```python
from build123d import *

# Parameters (mm, degrees)
SKETCH1_W           = 360
SKETCH1_H           = 210
BOSS_EXTRUDE1_DEPTH = 1
SKETCH2_R           = 5
SKETCH2_R_2         = 2.3
BOSS_EXTRUDE2_DEPTH = 5.7


with BuildPart() as part:
    # Sketch1 → Boss-Extrude1 (new body)
    with BuildSketch(Plane(origin=(0, 0, 0), x_dir=(1, 0, 0), z_dir=(0, 1, 0))):
        Rectangle(SKETCH1_W, SKETCH1_H)
        Polygon((28, -45.5), (0, -45.5), (0, 45.5), (-78.4, 45.5), (-78.4, -7.9), (-95, -7.9), (-95, 79.1), (-78.4, 79.1), (-78.4, 68.1), (28, 68.1), (28, 45.5), (66.5, 45.5), (66.5, -45.5), (66.5, -97), (28, -97), align=None, mode=Mode.SUBTRACT)
    extrude(amount=BOSS_EXTRUDE1_DEPTH)

    # Sketch2 → Boss-Extrude2 (add)
    with BuildSketch(Plane(origin=(0, 1, 0), x_dir=(1, 0, 0), z_dir=(0, 1, 0))):
        with Locations((-71.4, 75.1)):
            Circle(SKETCH2_R)
        with Locations((-71.4, 75.1)):
            Circle(SKETCH2_R_2, mode=Mode.SUBTRACT)
        with Locations((-71.4, 38.5)):
            Circle(SKETCH2_R)
        with Locations((-71.4, 38.5)):
            Circle(SKETCH2_R_2, mode=Mode.SUBTRACT)
        with Locations((-102, 75.1)):
            Circle(SKETCH2_R)
        with Locations((-102, 75.1)):
            Circle(SKETCH2_R_2, mode=Mode.SUBTRACT)
        with Locations((-7, 38.5)):
            Circle(SKETCH2_R)
        with Locations((-7, 38.5)):
            Circle(SKETCH2_R_2, mode=Mode.SUBTRACT)
        with Locations((35, 52.5)):
            Circle(SKETCH2_R)
        with Locations((35, 52.5)):
            Circle(SKETCH2_R_2, mode=Mode.SUBTRACT)
        with Locations((21, -52.5)):
            Circle(SKETCH2_R)
        with Locations((21, -52.5)):
            Circle(SKETCH2_R_2, mode=Mode.SUBTRACT)
        with Locations((-71.4, -0.9)):
            Circle(SKETCH2_R)
        with Locations((-71.4, -0.9)):
            Circle(SKETCH2_R_2, mode=Mode.SUBTRACT)
        with Locations((-102, -0.9)):
            Circle(SKETCH2_R)
        with Locations((-102, -0.9)):
            Circle(SKETCH2_R_2, mode=Mode.SUBTRACT)
        with Locations((73.5, 38.5)):
            Circle(SKETCH2_R)
        with Locations((73.5, 38.5)):
            Circle(SKETCH2_R_2, mode=Mode.SUBTRACT)
        with Locations((73.5, -90)):
            Circle(SKETCH2_R)
        with Locations((73.5, -90)):
            Circle(SKETCH2_R_2, mode=Mode.SUBTRACT)
        with Locations((21, -90)):
            Circle(SKETCH2_R)
        with Locations((21, -90)):
            Circle(SKETCH2_R_2, mode=Mode.SUBTRACT)
    extrude(amount=BOSS_EXTRUDE2_DEPTH)


solid = part.part
```
Model file for the job. Use its own axes, mm. A direction names the side the tool comes from. Round coordinates to 2 decimals unless told otherwise and drop trailing zeros. Write each loop counter-clockwise with the first axis right and the second up, starting at its lowest first coordinate (ties: lowest second). Pieces come first, ordered by that corner, then holes. Notation, with made-up numbers: (28, -23) -> (68, -23) arc R26 ccw to (68, -6) -> close; hole circle Ø2 at (-19.5, 63). An arc over 180 degrees is marked (long way). Answer as CSV lines item,"result".
1. Mould opens along X. For faces 3 (the face through (76.188, 3.81, -42.716)), 4 (the face through (-6, 6.7, -36)), 5 (the face through (31.315, 3.81, -55.879)) say: +X half, -X half, draft (parallel to the pull), parting line (faces both ways), or undercut.
Resolved:
face 3,"undercut"
face 4,"draft"
face 5,"parting line"
2. Tool access for faces 1 (the face through (-66.781, 3.81, 2.815)), 2 (the face through (76, 6.7, 91)): list every direction of +Z, -Z, +X, -X, +Y, -Y with a clear straight run to the whole face (end or side of a thin tool).
Resolved:
face 1,"+Y"
face 2,"+Z, -Z, +X, -X, +Y"
3. Drill centre lines: line 1 (Z direction, x = 73.5, y = 5.45); line 2 (X direction, y = 3.25, z = -38.5); line 3 (X direction, y = 2.8, z = -75.1). Where is each one in solid material? Low to high.
Resolved:
line 1,"-43.5 to -40.8, -36.2 to -33.5, 85 to 87.7, 92.3 to 95"
line 2,"-76.4 to -73.7, -69.1 to -66.4, -12 to -9.3, -4.7 to -2, 68.5 to 71.2, 75.8 to 78.5"
line 3,"-107 to -104.3, -99.7 to -97, -76.4 to -73.7, -69.1 to -66.4"
4. Slice it at A-A, the plane z = -63. List the corners of the cut face in (x, y), plus the area to 3 significant figures.
Resolved:
outline,"(-180, 0) -> (-95, 0) -> (-95, 1) -> (-180, 1) -> close; (28, 0) -> (180, 0) -> (180, 1) -> (28, 1) -> close"
area,"237 mm²"
5. Pin check, flat tips, straight feed: pin 1 Ø1 at (x, z) = (-110.5, 55.5) entering from +Y; pin 2 Ø2 at (y, z) = (2.5, 17.5) entering from +X; pin 3 Ø1.5 at (x, y) = (-67, 5) entering from -Z. Stop position of each tip, or through.
Resolved:
pin 1,"y = 1"
pin 2,"through"
pin 3,"z = -78.52"
6. Slice it at B-B, the plane y = 3.75. State how many separate pieces and enclosed holes the cut face has, plus the area to 3 significant figures.
Resolved:
separate pieces,"11"
enclosed holes,"11"
area,"681 mm²"
7. Slice it at C-C, the plane x = -17.5. List the corners of the cut face in (y, z), plus the area to 3 significant figures.
Resolved:
outline,"(0, -105) -> (1, -105) -> (1, -68.1) -> (0, -68.1) -> close; (0, -45.5) -> (1, -45.5) -> (1, 105) -> (0, 105) -> close"
area,"187 mm²"
